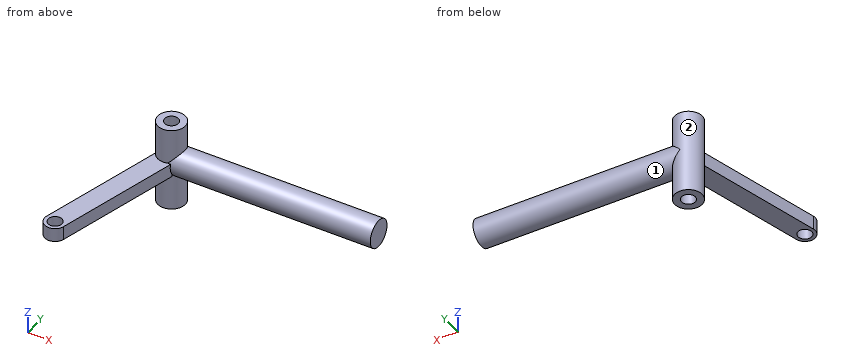
Solid Edge part; units mm, degrees
sketch "Sketch1" plane through (0, 0, 0) normal (0, -1, 0) x (1, 0, 0)
  line L0 (-10, -30.5) -> (0, -30.5)
  line L1 (0, 30.5) -> (0, -30.5)
  line L2 (0, 30.5) -> (-10, 30.5)
  line L3 (-10, 30.5) -> (-10, -30.5)
revolve "RevolvedProtrusion1" add sketch "Sketch1" angle 360 about axis through (0, 0, 54) along (0, 0, -1)
sketch "Sketch2" plane through (0, 0, 0) normal (1, 0, 0) x (0, 1, 0)
  circle A0 centre (0, 2) radius 10
extrude "Protrusion1" add sketch "Sketch2" along normal blind 150
sketch "Sketch3" plane through (0, 0, 0) normal (0, 0, 1) x (1, 0, 0)
  circle A0 centre (-25.8819, -96.5926) radius 5
  line L0 (-8.9564, -4.4479) -> (-33.1263, -94.6514)
  arc A1 (-33.1263, -94.6514) -> (-18.6375, -98.5337) centre (-25.8819, -96.5926) ccw
  line L1 (-18.6375, -98.5337) -> (5.5325, -8.3301)
  arc A2 (5.5325, -8.3301) -> (-8.9564, -4.4479) centre (0, 0) cw
  dimension "D1" = 33.1263
  dimension "D2" = 25.8819
extrude "Styrarm" add sketch "Sketch3" along normal mid plane 10
hole "Hole1" at (0, 0, 30.5) direction (0, 0, -1) diameter 10 end up to next
Input: part model. Units: mm. Frame: model coordinates. Face numbers are marked on the shaded views. A direction names the side the tool comes from. Round coordinates to 2 decimals unless told otherwise and drop trailing zeros. Loops run counter-clockwise (first coordinate to the right, second up) from the corner with the lowest first, then second, coordinate; pieces in that order, holes last. Notation, with made-up numbers: (3, 60) -> (53, 60) arc R23 cw to (53, 71) -> close; hole circle Ø7 at (84, 43). An arc over 180 degrees is marked (long way). One line per item, written item: value.
(1) Section A-A (y = 0). Return the cut outline in (x, z), plus the area to 3 significant figures.
Geometry check:
outline: (-10, -30.5) -> (-5, -30.5) -> (-5, 30.5) -> (-10, 30.5) -> close; (5, -30.5) -> (10, -30.5) -> (10, -8) -> (150, -8) -> (150, 12) -> (10, 12) -> (10, 30.5) -> (5, 30.5) -> close
area: 3,410 mm2
(2) Section C-C (x = 122.5). Return the cut outline in (y, z).
Geometry check:
outline: circle Ø20 at (0, 2)
(3) Section D-D (z = 25). Return the cut outline in (x, y), plus the area to 3 significant figures.
Geometry check:
outline: circle Ø20 at (0, 0); hole circle Ø10 at (0, 0)
area: 236 mm2
(4) Set-up query: the marked faces 1 and 2. Return all of +Z, -Z, +X, -X, +Y, -Y with unobstructed straight access to the full face (end or side cutting, diameter ignored); none if empty.
Geometry check:
face 1: +X
face 2: none
(5) Section B-B (z = 2). Return the cut outline in (x, y), plus the area to 3 significant figures.
Geometry check:
outline: (-33.13, -94.65) arc R7.5 ccw to (-18.64, -98.53) -> (5.09, -10) -> (150, -10) -> (150, 10) -> (0, 10) arc R10 ccw to (-8.96, -4.45) -> close; hole circle Ø10 at (-25.88, -96.59); hole circle Ø10 at (0, 0)
area: 4,450 mm2
(6) Pin query (flat end, axial travel): pin 1 (11.5 mm diameter, centred on x = -12, y = -75, fed in from +Z); pin 2 (8 mm diameter, centred on y = -43, z = -3, fed in from +X); pin 3 (10 mm diameter, centred on x = 51, z = 15, fed in from +Y). Return the tip coordinate at first contact, or that it passes through.
Geometry check:
pin 1: z = 5
pin 2: x = -2.69
pin 3: y = 6
(7) Material intervals for line 1 (Y direction, x = 0, z = 18); line 2 (Z direction, x = 20, y = -0.5); line 3 (X direction, y = 2, z = -2.5), sorted ascending. Write a range as [from, to].
Geometry check:
line 1: [-10, -5], [5, 10]
line 2: [-7.99, 11.99]
line 3: [-9.8, -4.58], [4.58, 150]
